```python
from build123d import *

# Parameters (mm, degrees)
F0_W     = 6.096
F0_H     = 6.35
F2_R     = 5.08
F3_DEPTH = 24.13
F4_R     = 2.54
F5_W     = 2.032
F5_H     = 2.54
F6_DEPTH = 24.13


with BuildPart() as f1:
    # F0 (on Front) → F1 (revolve)
    with BuildSketch(Plane.XZ):
        Polygon((0, 19.05), (0, 0), (19.05, 0), (19.05, 2.032), (17.018, 2.032), (6.096, 19.05), align=None)
        with Locations((3.048, 22.225)):
            Rectangle(F0_W, F0_H)
    revolve(axis=Axis((0, 0, 9.525), (0, 0, 1)))

    # F2 (on face) → F3 (join)
    with BuildSketch(Plane.XY.offset(25.4)):
        Circle(F2_R)
    extrude(amount=F3_DEPTH)

    # F4
    f4_edges = [f1.edges().sort_by_distance(p)[0] for p in [
        (-6.096, 0, 19.05),
    ]]
    fillet(f4_edges, radius=F4_R)

    # F5 (on face) → F6 (cut)
    with BuildSketch(Plane.XY.offset(49.53)):
        with Locations((0, 4.318)):
            Rectangle(F5_W, F5_H)
        with Locations((0, -4.318)):
            Rectangle(F5_W, F5_H)
    extrude(amount=-F6_DEPTH, mode=Mode.SUBTRACT)


solid = f1.part
```
Design review of the part built by this model. Coordinates are the model's own, in mm. A direction names the side the tool comes from. Give positions to 0.01 mm unless a question says otherwise; leave off trailing zeros. Write each loop counter-clockwise with the first axis right and the second up, starting at its lowest first coordinate (ties: lowest second). Pieces come first, ordered by that corner, then holes.
(1) Clearance check with flat-ended pins moving along their axes: pin 1 Ø12 at (y, z) = (15, 19) entering from -X; pin 2 Ø0.6 at (y, z) = (-4, 42) entering from +X; pin 3 Ø11.5 at (x, y) = (4.5, 4.5) entering from +Z; pin 4 Ø2 at (y, z) = (-3.5, 34) entering from -X. State where each tip first meets the part, or that it passes through.
Checked values:
pin 1: passes through
pin 2: stops at x = 3.48
pin 3: stops at z = 49.53
pin 4: stops at x = -4.42
(2) Tool access review of faces 1 (the face through (0, -3.048, 38)), 2 (the face through (-7, 16, 2.032)), 3 (the face through (-1.016, 4, 38)), 4 (the face through (-5.08, 0.1, 37.3)), 5 (the face through (5.08, -0.1, 37.3)): name each direction out of +Z, -Z, +X, -X, +Y, -Y from which nothing blocks a thin tool from reaching the whole face with its end or side.
Checked values:
face 1: +Z, -Y
face 2: +Z
face 3: +Z, +Y
face 4: +Z, -X
face 5: +Z, +X
(3) Add section B-B (z = 14). Give the boundary of the cut face in (x, y), and give its area (3 significant figures).
Checked values:
outline: circle Ø18.67 at (0, 0)
area: 274 mm2
(4) Mouldability with a two-part tool opening along X and no side actions: class faces 6 (the face through (0, 3.048, 38)), 7 (the face through (-1.77, -7.98, 15.81)), 8 (the face through (0, 0, 0)), 9 (the face through (-1.016, -4, 38)) as +X half, -X half, draft (parallel to the pull), parting line (faces both ways), or undercut.
Checked values:
face 6: undercut
face 7: parting line
face 8: draft
face 9: undercut
(5) Add section A-A (z = 31.5). Give the boundary of the cut face in (x, y), and give its area (3 significant figures).
Checked values:
outline: (-1.02, -4.98) - (-1.02, -3.05) - (1.02, -3.05) - (1.02, -4.98) arc R5.08 ccw to (1.02, 4.98) - (1.02, 3.05) - (-1.02, 3.05) - (-1.02, 4.98) arc R5.08 ccw to start
area: 73.0 mm2
(6) Wall thickness on line 1 along Z through (x, y) = (-14, 12.5); line 2 along X through (y, z) = (4, 34); line 3 along Y through (x, z) = (-3.5, 22.5): over which ranges is each line inside the solid? List them lowest first.
Checked values:
line 1: z = 0 to 2.03
line 2: x = -3.13 to -1.02, 1.02 to 3.13
line 3: y = -4.99 to 4.99
